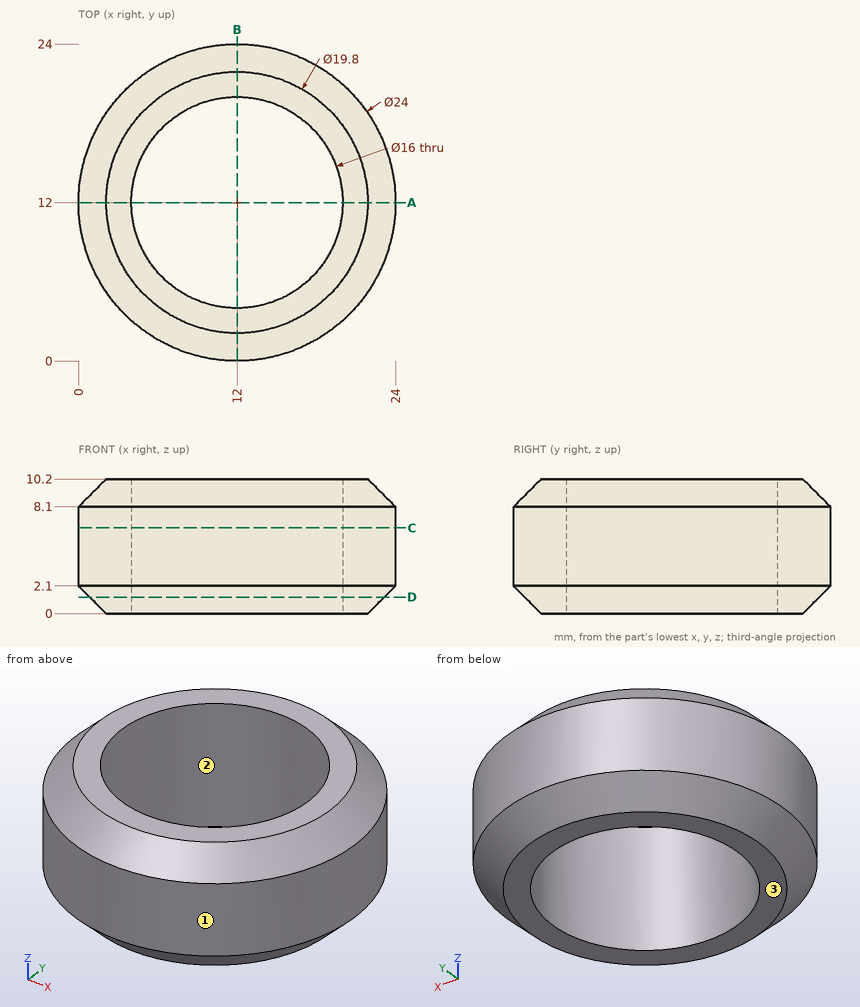
Check sheet for the drawn part. Datum: minimum x, y, z corner. Units: mm. Round coordinates to 2 decimals unless told otherwise and drop trailing zeros. Order: outer loops, then holes, each group sorted by start corner. A loop starts at its lowest first (then second) coordinate and runs counter-clockwise, first axis right, second up.
1. Release check for a two-part mould opening along Y. For the marked faces 1, 2 and 3 record: +Y half, -Y half, draft (parallel to the pull), parting line (faces both ways), or undercut.
Final values:
face 1: parting line
face 2: undercut
face 3: draft
2. Section check A-A on y = 12. Record the cut outline in (x, z), then the cut area to 3 significant figures.
Final values:
outline: (0, 2.1) - (2.1, 0) - (4, 0) - (4, 10.2) - (2.1, 10.2) - (0, 8.1) - close; (20, 0) - (21.9, 0) - (24, 2.1) - (24, 8.1) - (21.9, 10.2) - (20, 10.2) - close
area: 72.8 mm2
3. Section check C-C on z = 6.5. Record the cut outline in (x, y).
Final values:
outline: circle Ø24 at (12, 12); hole circle Ø16 at (12, 12)
4. Go/stop test with flat-tipped pins: P1, Ø1, axis at x = 3, z = 8.5, coming from the -Y side (3 decimals); P2, Ø3, axis at x = 3.5, y = 12, coming from the -Z side; P3, Ø3, axis at y = 19.5, z = 4, coming from the +X side; P4, Ø4, axis at x = 8, y = 15, coming from the +Z side. Record where each tip stops, or that it passes through.
Final values:
P1: stops at y = 3.735
P2: stops at z = 0
P3: stops at x = 22.39
P4: passes through
5. Section check D-D on z = 1.25. Record the cut outline in (x, y).
Final values:
outline: circle Ø22.3 at (12, 12); hole circle Ø16 at (12, 12)
6. Thickness scan on L1, parallel to X at y = 12, z = 6.25; L2, parallel to X at y = 9, z = 2.75. Record the ranges inside material, lowest first.
Final values:
L1: x = 0 to 4, 20 to 24
L2: x = 0.38 to 4.58, 19.42 to 23.62
